For this review, take the finished solid that the model builds, in its own axes (mm). A direction names the side the tool comes from. Round coordinates to 2 decimals unless told otherwise and drop trailing zeros. Write each loop counter-clockwise with the first axis right and the second up, starting at its lowest first coordinate (ties: lowest second). Pieces come first, ordered by that corner, then holes.
from build123d import *

# Parameters (mm, degrees)
SKETCH3_R           = 6
BOSS_EXTRUDE1_DEPTH = 6
SKETCH4_R           = 3
BOSS_EXTRUDE2_DEPTH = 3.5
BOSS_EXTRUDE3_DEPTH = 12
SKETCH6_R           = 0.25
BOSS_EXTRUDE4_DEPTH = 8


with BuildPart() as part:
    # Sketch2 → Revolve1 (revolve)
    with BuildSketch(Plane.XY):
        Polygon((88, 0), (88, 18.5), (65, 18.5), (65, 16.5), (53, 16.5), (53, 18.5), (20, 18.5), (20, 16.5), (8, 16.5), (8, 8), (4, 8), (4, 2), (0, 2), (0, 0), align=None)
    revolve(axis=Axis((88, 0, 0), (-1, 0, 0)))

    # Sketch3 → Boss-Extrude1 (add)
    with BuildSketch(Plane(origin=(88, 0, 0), x_dir=(0, 0, -1), z_dir=(1, 0, 0))):
        with Locations((0, 11.056321537)):
            Circle(SKETCH3_R)
    extrude(amount=BOSS_EXTRUDE1_DEPTH)

    # Sketch4 → Boss-Extrude2 (add)
    with BuildSketch(Plane(origin=(94, 0, 0), x_dir=(0, 0, -1), z_dir=(1, 0, 0))):
        with Locations((0, 11.056321537)):
            Circle(SKETCH4_R)
    extrude(amount=BOSS_EXTRUDE2_DEPTH)

    # Sketch5 → Boss-Extrude3 (add)
    with BuildSketch(Plane(origin=(97.5, 0, 0), x_dir=(0, 0, -1), z_dir=(1, 0, 0))):
        with BuildLine():
            Line((1.658312395, 8.556321537), (-1.658312395, 8.556321537))
            ThreePointArc((-1.658312395, 8.556321537), (0, 14.056321537), (1.658312395, 8.556321537))
        make_face()
    extrude(amount=BOSS_EXTRUDE3_DEPTH)

    # Sketch6 → Boss-Extrude4 (add)
    with BuildSketch(Plane.ZY.offset(-8)):
        with Locations((0, 14)):
            Circle(SKETCH6_R)
        with Locations((12.124355653, -7)):
            Circle(SKETCH6_R)
        with Locations((-12.124355653, -7)):
            Circle(SKETCH6_R)
    extrude(amount=BOSS_EXTRUDE4_DEPTH)


solid = part.part
(1) For pin 1 Ø16.5 at (y, z) = (-6.5, 6.5) entering from -X; pin 2 Ø11 at (y, z) = (-0.5, 2.5) entering from +X; pin 3 Ø3 at (x, z) = (65.5, 6) entering from -Y; pin 4 Ø1.7 at (x, z) = (101, 0) entering from -Y, all flat-tipped, find the tip position at first contact; note any pin that passes through.
Geometry check:
pin 1: stops at x = 0
pin 2: stops at x = 88
pin 3: stops at y = -17.94
pin 4: stops at y = 8.56
(2) We need section B-B, the plane z = 4.5. Give the boundary of the cut face in (x, y).
Geometry check:
outline: (4, -6.61) - (8, -6.61) - (8, -15.87) - (20, -15.87) - (20, -17.94) - (53, -17.94) - (53, -15.87) - (65, -15.87) - (65, -17.94) - (88, -17.94) - (88, 7.09) - (94, 7.09) - (94, 15.02) - (88, 15.02) - (88, 17.94) - (65, 17.94) - (65, 15.87) - (53, 15.87) - (53, 17.94) - (20, 17.94) - (20, 15.87) - (8, 15.87) - (8, 6.61) - (4, 6.61) - close
(3) We need section D-D, the plane y = -11. Give the boundary of the cut face in (x, z).
Geometry check:
outline: (8, -12.3) - (20, -12.3) - (20, -14.87) - (53, -14.87) - (53, -12.3) - (65, -12.3) - (65, -14.87) - (88, -14.87) - (88, 14.87) - (65, 14.87) - (65, 12.3) - (53, 12.3) - (53, 14.87) - (20, 14.87) - (20, 12.3) - (8, 12.3) - close
(4) For faces 5 (the face through (91, 5.2, 1.3)), 6 (the face through (58.92, 15.24, 6.32)), 7 (the face through (103, 8.556, 0)), 8 (the face through (2, 0, 2)), list the 3-axis set-ups (+Z, -Z, +X, -X, +Y, -Y) from which the entire face can be reached by the end or side of a thin tool; tool diameter is ignored.
Geometry check:
face 5: +X
face 6: none
face 7: +Z, -Z, +X, -Y
face 8: -X
(5) We need section C-C, the plane x = 45.5. Give the boundary of the cut face in (y, z), and give its area (3 significant figures).
Geometry check:
outline: circle Ø37 at (0, 0)
area: 1,080 mm2
(6) Mouldability with a two-part tool opening along X and no side actions: class faces 1 (the face through (53, 17, 0)), 2 (the face through (94, 10, 3)), 3 (the face through (65, -17, 0)), 4 (the face through (5.97, -1.73, 7.81)) as pulls with the +X half, pulls with the -X half, needs draft (parallel to the pull), parting line crosses it, or undercut.
Geometry check:
face 1: undercut
face 2: pulls with the +X half
face 3: undercut
face 4: needs draft
(7) We need section A-A, the plane y = 0. Give the boundary of the cut face in (x, z), and give its area (3 significant figures).
Geometry check:
outline: (0, -2) - (4, -2) - (4, -8) - (8, -8) - (8, -16.5) - (20, -16.5) - (20, -18.5) - (53, -18.5) - (53, -16.5) - (65, -16.5) - (65, -18.5) - (88, -18.5) - (88, 18.5) - (65, 18.5) - (65, 16.5) - (53, 16.5) - (53, 18.5) - (20, 18.5) - (20, 16.5) - (8, 16.5) - (8, 8) - (4, 8) - (4, 2) - (0, 2) - close
area: 2,940 mm2
(8) For line 1 along X through (y, z) = (7, -15); line 2 along X through (y, z) = (-9, 5.5); line 3 along Z through (x, y) = (80.5, -0.5), list the stretches that pass through material, from the lowest coordinate up.
Geometry check:
line 1: x = 20 to 53, 65 to 88
line 2: x = 8 to 88
line 3: z = -18.49 to 18.49
